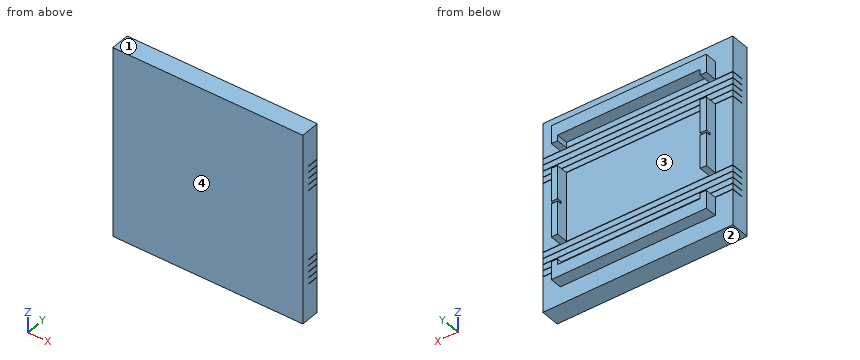
Autodesk Inventor part; units mm, degrees
ref_plane "YZ Plane" through (0, 0, 0) normal (1, 0, 0) x (0, 1, 0)
ref_plane "XZ Plane" through (0, 0, 0) normal (0, 1, 0) x (-1, 0, 0)
ref_plane "XY Plane" through (0, 0, 0) normal (0, 0, 1) x (1, 0, 0)
sketch "Boceto1" plane through (0, 0, 0) normal (0, 1, 0) x (-1, 0, 0)
  line L0 (0, 0) -> (80, 0)
  line L1 (80, 0) -> (80, -80)
  line L2 (80, -80) -> (0, -80)
  line L3 (0, -80) -> (0, 0)
  line L4 (10, -70) -> (70, -70)
  line L5 (70, -70) -> (70, -10)
  line L6 (70, -10) -> (10, -10)
  line L7 (10, -10) -> (10, -70)
  line L8 (0, -12.375) -> (80, -12.375)
  line L9 (0, -14.95) -> (80, -14.95)
  line L10 (0, -17.525) -> (80, -17.525)
  line L11 (80, -20.1) -> (0, -20.1)
  line L12 (0, -22.675) -> (80, -22.675)
  line L13 (0, -12.575) -> (80, -12.575)
  line L14 (0, -15.15) -> (80, -15.15)
  line L15 (0, -17.725) -> (80, -17.725)
  line L16 (80, -20.3) -> (0, -20.3)
  line L17 (0, -22.875) -> (80, -22.875)
  line L18 (0, -25.25) -> (80, -25.25)
  line L19 (0, -25.45) -> (80, -25.45)
  line L20 (10, -40) -> (80, -40)
  line L21 (0, -67.625) -> (80, -67.625)
  line L22 (0, -65.05) -> (80, -65.05)
  line L23 (0, -62.475) -> (80, -62.475)
  line L24 (80, -59.9) -> (0, -59.9)
  line L25 (0, -57.325) -> (80, -57.325)
  line L26 (0, -67.425) -> (80, -67.425)
  line L27 (0, -64.85) -> (80, -64.85)
  line L28 (0, -62.275) -> (80, -62.275)
  line L29 (80, -59.7) -> (0, -59.7)
  line L30 (0, -57.125) -> (80, -57.125)
  line L31 (0, -54.75) -> (80, -54.75)
  line L32 (0, -54.55) -> (80, -54.55)
  line L33 (72.625, -7.375) -> (7.375, -7.375)
  line L34 (7.375, -7.375) -> (7.375, -72.625)
  line L35 (7.375, -72.625) -> (72.625, -72.625)
  line L36 (72.625, -72.625) -> (72.625, -7.375)
  line L37 (7.375, 0) -> (0, 0)
  line L38 (7.375, -80) -> (0, -80)
  point P0 (10, -12.375)
  point P1 (70, -12.375)
  point P2 (10, -14.95)
  point P3 (70, -14.95)
  point P4 (10, -17.525)
  point P5 (70, -17.525)
  point P6 (70, -20.1)
  point P7 (10, -20.1)
  point P8 (10, -22.675)
  point P9 (70, -22.675)
  point P10 (10, -12.575)
  point P11 (70, -12.575)
  point P12 (10, -15.15)
  point P13 (70, -15.15)
  point P14 (10, -17.725)
  point P15 (70, -17.725)
  point P16 (70, -20.3)
  point P17 (10, -20.3)
  point P18 (10, -22.875)
  point P19 (70, -22.875)
  point P20 (10, -25.25)
  point P21 (70, -25.25)
  point P22 (10, -25.45)
  point P23 (70, -25.45)
  point P24 (10, -67.625)
  point P25 (70, -67.625)
  point P26 (10, -65.05)
  point P27 (70, -65.05)
  point P28 (10, -62.475)
  point P29 (70, -62.475)
  point P30 (70, -59.9)
  point P31 (10, -59.9)
  point P32 (10, -57.325)
  point P33 (70, -57.325)
  point P34 (10, -67.425)
  point P35 (70, -67.425)
  point P36 (10, -64.85)
  point P37 (70, -64.85)
  point P38 (10, -62.275)
  point P39 (70, -62.275)
  point P40 (70, -59.7)
  point P41 (10, -59.7)
  point P42 (10, -57.125)
  point P43 (70, -57.125)
  point P44 (10, -54.75)
  point P45 (70, -54.75)
  point P46 (10, -54.55)
  point P47 (70, -54.55)
  point P48 (72.625, -12.375)
  point P49 (7.375, -12.375)
  point P50 (72.625, -54.55)
  point P51 (72.625, -25.45)
  point P52 (70, -25.45)
  point P53 (70, -54.55)
  point P54 (7.375, -25.45)
  point P55 (7.375, -54.55)
  point P56 (10, -54.55)
  point P57 (10, -25.45)
  point P58 (10, -67.625)
  point P59 (7.375, -67.625)
  point P60 (72.625, -67.625)
  point P61 (70, -67.625)
  point P62 (7.375, -14.95)
  point P63 (72.625, -14.95)
  point P64 (72.625, -65.05)
  point P65 (70, -65.05)
  point P66 (10, -65.05)
  point P67 (7.375, -65.05)
  point P68 (70, -67.425)
  point P69 (10, -67.425)
  point P70 (10, -12.575)
  point P71 (70, -12.575)
  dimension "d0" = 80
  dimension "d1" = 80
  dimension "d2" = 60
  dimension "d3" = 60
  dimension "d4" = 10
  dimension "d5" = 10
  dimension "d6" = 2.375
  dimension "d7" = 0.2
  dimension "d8" = 2.375
  dimension "d9" = 0.2
  dimension "d10" = 0.2
  dimension "d11" = 0.2
  dimension "d12" = 0.2
  dimension "d13" = 2.375
  dimension "d14" = 2.375
  dimension "d15" = 2.375
  dimension "d16" = 2.375
  dimension "d17" = 0.2
  dimension "d35" = 5
extrude "Extrusión1" add sketch "Boceto1" along normal blind 5 contours L0 L1 L8 L36 L33 L34 L3 | L8 L34 L13 L3 | L13 L34 L9 L3 | L34 L33 L36 L8 L5 L6 L7 | L8 L7 L13 L34 | L1 L13 L36 L8 | L13 L7 L9 L34 | L8 L5 L13 L7 | L7 L6 L5 L8 | L1 L9 L36 L13 | L36 L13 L5 L8 | L14 L34 L10 L3 | L13 L5 L9 L7 | L36 L9 L5 L13 | L14 L7 L10 L34 | L1 L10 L36 L14 | L15 L34 L11 L3 | L14 L5 L10 L7 | L36 L10 L5 L14 | L15 L7 L11 L34 | L1 L11 L36 L15 | L16 L34 L12 L3 | L15 L5 L11 L7 | L36 L11 L5 L15 | L16 L7 L12 L34 | L1 L12 L36 L16 | L17 L34 L18 L3 | L16 L5 L12 L7 | L36 L12 L5 L16 | L17 L7 L18 L34 | L1 L18 L36 L17 | L19 L34 L32 L3 | L17 L5 L18 L7 | L36 L18 L5 L17 | L19 L7 L32 L34 | L1 L20 L36 L19 | L31 L34 L30 L3 | L19 L5 L20 L7 | L1 L32 L36 L20 | L36 L20 L5 L19 | L31 L7 L30 L34 | L7 L20 L5 L32 | L36 L32 L5 L20 | L25 L34 L29 L3 | L31 L5 L30 L7 | L1 L30 L36 L31 | L25 L7 L29 L34 | L31 L36 L30 L5 | L24 L34 L28 L3 | L25 L5 L29 L7 | L1 L29 L36 L25 | L24 L7 L28 L34 | L25 L36 L29 L5 | L23 L34 L27 L3 | L24 L5 L28 L7 | L1 L28 L36 L24 | L23 L7 L27 L34 | L24 L36 L28 L5 | L22 L34 L26 L3 | L23 L5 L27 L7 | L1 L27 L36 L23 | L26 L34 L21 L3 | L22 L7 L26 L34 | L23 L36 L27 L5 | L21 L34 L35 L36 L1 L2 L3 | L26 L7 L21 L34 | L22 L5 L26 L7 | L1 L26 L36 L22 | L21 L7 L4 L5 L36 L35 L34 | L26 L5 L21 L7 | L22 L36 L26 L5 | L1 L21 L36 L26 | L21 L5 L4 L7 | L26 L36 L21 L5
sketch "Boceto2" plane through (0, 0, 0) normal (0, -1, 0) x (1, 0, 0)
  line L0 (0, -80) -> (-80, -80)
  line L1 (-80, 0) -> (0, 0)
  line L2 (-80, -80) -> (-80, 0)
  line L3 (-80, 0) -> (0, 0)
  line L4 (-80, -65.05) -> (0, -65.05) construction
  line L5 (0, 0) -> (0, -80)
  line L6 (-80, -80) -> (0, -80)
extrude "Extrusión4" add sketch "Boceto2" along normal blind 3
extrude "Extrusión5" add sketch "Boceto1" along normal blind 10 contours L34 L33 L36 L8 L5 L6 L7 | L8 L7 L13 L34 | L13 L7 L9 L34 | L8 L5 L13 L7 | L7 L6 L5 L8 | L36 L13 L5 L8 | L36 L9 L5 L13 | L19 L7 L32 L34 | L36 L20 L5 L19 | L36 L32 L5 L20 | L22 L7 L26 L34 | L26 L7 L21 L34 | L21 L7 L4 L5 L36 L35 L34 | L26 L5 L21 L7 | L22 L36 L26 L5 | L21 L5 L4 L7 | L26 L36 L21 L5
sketch "Boceto3" plane through (0, 10, 0) normal (0, 1, 0) x (1, 0, 0)
  line L0 (-7.375, 25.45) -> (-7.375, 54.55)
  line L1 (-7.375, 40) -> (-86.5517, 40)
  line L2 (-5, 39.5) -> (-84.1767, 39.5)
  line L3 (-5, 40.5) -> (-84.1767, 40.5)
  line L4 (-10, 54.55) -> (-10, 25.45)
  line L5 (-5, 40.5) -> (-5, 39.5)
  line L6 (-84.1767, 40.5) -> (-84.1767, 39.5)
  point P0 (0, 0)
  point P1 (-10, 40)
  point P2 (-10, 39.5)
  point P3 (-10, 40.5)
  point P4 (-7.375, 39.5)
  point P5 (-7.375, 40.5)
  dimension "d31" = 0.5
  dimension "d32" = 0.5
extrude "Extrusión6" cut sketch "Boceto3" against normal blind 2 contours L2 L4 L1 L0 | L1 L4 L3 L0 | L2 L6 L1 L4 | L1 L6 L3 L4
equation "\"d8\" = d6"
equation "\"d9\" = d7"
equation "\"d10\" = d9"
equation "\"d11\" = d7"
equation "\"d12\" = d7"
equation "\"d13\" = d6"
equation "\"d14\" = d6"
equation "\"d15\" = d6"
equation "\"d16\" = d6"
equation "\"d17\" = d7"
properties part number "Cortador Ancho PDMS5.5"
CAD build for the part. Positions are in the model's coordinates, mm. Face numbers are marked on the shaded views. Coordinates: 2 decimals unless noted, no trailing zeros. Write each loop counter-clockwise with the first axis right and the second up, starting at its lowest first coordinate (ties: lowest second). Pieces come first, ordered by that corner, then holes. Notation, with made-up numbers: (83, 1) -> (114, 1) arc R16 ccw to (114, 10) -> close; hole circle Ø7 at (-24, -31.5). An arc over 180 degrees is marked (long way). Use CSV: the item, a comma, the result in double quotes. Start each with the question number.
Item 1: Drop flat-ended pins along their axis: P1, Ø1.5, axis at y = 8.5, z = -70, coming from the +X side (3 decimals); P2, Ø2, axis at x = -71, y = 8.5, coming from the -Z side (3 decimals); P3, Ø1.9, axis at x = -36.5, z = -66, coming from the +Y side. Give the stop position or say it passes through.
Item 2: Band-saw the part on B-B, the plane y = 4. Give the number of separate pieces and of enclosed holes in the cut face, plus the area to 3 significant figures.
Item 3: Two-plate mould, pull along Z, no slides. Class the marked faces 1, 2, 3 and 4: +Z half, -Z half, draft (parallel to the pull), parting line (faces both ways), or undercut.
Item 4: Wall check: probe 1 along Z at (x, y) = (-9, 9.25) (3 decimals); probe 2 along X at (y, z) = (6, -38) (3 decimals); probe 3 along Z at (x, y) = (-48, 6) (3 decimals). Give the ranges that are in metal, low to high.
Item 5: Band-saw the part on A-A, the plane z = -50.5. Write the cut outline in (x, y) (3 decimals).
Response values:
1,P1,"stops at x = -7.375"
1,P2,"stops at z = -72.625"
1,P3,"stops at y = 5"
2,separate pieces,"11"
2,enclosed holes,"0"
2,area,"6,240 mm2"
3,face 1,"+Z half"
3,face 2,"-Z half"
3,face 3,"undercut"
3,face 4,"draft"
4,probe 1,"z = -72.625 to -65.05, -54.55 to -40.5, -39.5 to -25.45, -14.95 to -7.375"
4,probe 2,"x = -72.625 to -70, -10 to -7.375"
4,probe 3,"z = -72.625 to -67.425, -12.575 to -7.375"
5,outline,"(-80, -3) -> (0, -3) -> (0, 5) -> (-7.375, 5) -> (-7.375, 10) -> (-10, 10) -> (-10, 5) -> (-70, 5) -> (-70, 10) -> (-72.625, 10) -> (-72.625, 5) -> (-80, 5) -> close"
